Geometry: final body of the model. Coordinates: model frame, mm. A direction names the side the tool comes from. Give positions to 0.01 mm unless a question says otherwise; leave off trailing zeros. Loops run counter-clockwise (first coordinate to the right, second up) from the corner with the lowest first, then second, coordinate; pieces in that order, holes last. Notation, with made-up numbers: M 30.25,15 L 35.25,15 A35 ccw 35.25,47 Z; hole C 19,-4 d9. An arc over 180 degrees is marked long. Put each result on its own line as item: value.
```python
from build123d import *

# Parameters (mm, degrees)
SKETCH1_W           = 40
SKETCH1_H           = 8
SKETCH1_R           = 2.5
BOSS_EXTRUDE1_DEPTH = 3


with BuildPart() as part:
    # Sketch1 → Boss-Extrude1 (new body)
    with BuildSketch(Plane.XY):
        with Locations((0.003679189, 1.000819415)):
            Rectangle(SKETCH1_W, SKETCH1_H)
        with BuildLine():
            Line((-8.246320143, 3.165882539), (-6.746321478, 2.29985729))
            ThreePointArc((-6.746321478, 2.29985729), (-5.996321879, 1.000819415), (-6.746321478, -0.298218459))
            Line((-6.746321478, -0.298218459), (-8.246320143, -1.164243709))
            ThreePointArc((-8.246320143, -1.164243709), (-10.636363972, -1.224107908), (-11.983789404, 0.750819415))
            ThreePointArc((-11.983789404, 0.750819415), (-11.996320811, 1.000819415), (-11.983789404, 1.250819415))
            ThreePointArc((-11.983789404, 1.250819415), (-10.636363972, 3.225746738), (-8.246320143, 3.165882539))
        make_face(mode=Mode.SUBTRACT)
        with Locations((0.003679189, 1.000819415)):
            Circle(SKETCH1_R, mode=Mode.SUBTRACT)
        with BuildLine():
            Line((8.244905291, 3.163423753), (8.247736867, 3.165063509))
            ThreePointArc((8.247736867, 3.165063509), (10.638467861, 3.226118523), (11.986620451, 1.250819308))
            ThreePointArc((11.986620451, 1.250819308), (11.999151848, 1.000819415), (11.986620451, 0.750819522))
            ThreePointArc((11.986620451, 0.750819522), (10.637740693, -1.224851841), (8.246322819, -1.162606427))
            Line((8.246322819, -1.162606427), (6.751978531, -0.297235948))
            ThreePointArc((6.751978531, -0.297235948), (6.003678121, 1.000819415), (6.751978531, 2.298874779))
            Line((6.751978531, 2.298874779), (8.244905291, 3.163423753))
        make_face(mode=Mode.SUBTRACT)
    extrude(amount=BOSS_EXTRUDE1_DEPTH)


solid = part.part
```
Item 1: Pin query (flat end, axial travel): pin 1 Ø2 at (x, y) = (-8.5, 0.5) entering from -Z. Return the tip coordinate at first contact, or that it passes through.
Output values:
pin 1: through
Item 2: Section B-B on z = 0.9. Output: boundary loops of the cut face in (x, y).
Output values:
outline: M -20,-3 L 20,-3 L 20,5 L -20,5 Z; hole M -8.25,-1.16 L -6.75,-0.3 A1.5 ccw -6.75,2.3 L -8.25,3.17 A2.5 ccw long Z; hole C 0,1 d5; hole M 6.75,-0.3 L 8.25,-1.16 A2.5 ccw long 8.25,3.17 L 6.75,2.3 A1.5 ccw Z
Item 3: Section A-A on x = -10. Output: boundary loops of the cut face in (y, z), then the cut area to 3 significant figures.
Output values:
outline: M -3,0 L -1.45,0 L -1.45,3 L -3,3 Z; M 3.45,0 L 5,0 L 5,3 L 3.45,3 Z
area: 9.31 mm²
Item 4: Set-up query: faces 4 (the flat face through (-7.486, -0.725, 1.479)), 5 (the flat face through (0, 5.001, 1)). Return all of +Z, -Z, +X, -X, +Y, -Y with unobstructed straight access to the full face (end or side cutting, diameter ignored); none if empty.
Output values:
face 4: +Z, -Z
face 5: +Z, -Z, +X, -X, +Y
Item 5: Mould query, pull axis Y, two halves, no side actions, for faces 1 (the flat face through (0, -2.999, 1)), 2 (the cylindrical face through (-5.996, 1.023, 1.479)), 3 (the flat face through (0, 4, 3)). Classes: pulls with the +Y half, pulls with the -Y half, needs draft (parallel to the pull), parting line crosses it, or undercut.
Output values:
face 1: pulls with the -Y half
face 2: undercut
face 3: needs draft
Item 6: Line query: probe 1 along X at (y, z) = (1.25, 2.55); probe 2 along X at (y, z) = (2, 1.15); probe 3 along Y at (x, z) = (10.5, 2.2). Output: solid intervals per line, ascending. Write a range as [from, to].
Output values:
probe 1: [-20, -11.98], [-6.02, -2.48], [2.49, 6.02], [11.99, 20]
probe 2: [-20, -11.79], [-6.38, -2.29], [2.3, 6.38], [11.79, 20]
probe 3: [-3, -1.29], [3.29, 5]
